CAD build for the part. Positions are in the model's coordinates, mm. A direction names the side the tool comes from. Give positions to 0.01 mm unless a question says otherwise; leave off trailing zeros. Write each loop counter-clockwise with the first axis right and the second up, starting at its lowest first coordinate (ties: lowest second). Pieces come first, ordered by that corner, then holes. Notation, with made-up numbers: (-27.5, 61) - (11.5, 61) arc R22 cw to (11.5, 69) - close; hole circle Ø9 at (16, 21.25). An arc over 180 degrees is marked (long way). Answer as a JSON object with one key per item and string values.
from build123d import *

# Parameters (mm, degrees)
SKETCH1_R           = 1.5
SKETCH1_R_2         = 6.25
SKETCH1_R_3         = 2.55
SKETCH1_R_4         = 4.25
BOSS_EXTRUDE1_DEPTH = 12
SKETCH2_R           = 9
CUT_EXTRUDE1_DEPTH  = 2
SKETCH3_R           = 1.5
CUT_EXTRUDE2_DEPTH  = 210.485083001
SKETCH4_R           = 3.25
CUT_EXTRUDE3_DEPTH  = 25
FILLET1_R           = 2


with BuildPart() as part:
    # Sketch1 → Boss-Extrude1 (new body)
    with BuildSketch(Plane(origin=(0, 0, 0), x_dir=(1, 0, 0), z_dir=(0, 1, 0))):
        with BuildLine():
            Line((55, 122), (55, 117))
            Line((55, 117), (0, 117))
            Line((0, 117), (0, 0))
            Line((0, 0), (30, 0))
            Line((30, 0), (30, 1))
            Line((30, 1), (72.5, 1))
            Line((72.5, 1), (72.5, -39))
            Line((72.5, -39), (82.5, -39))
            Line((82.5, -39), (82.5, 40))
            ThreePointArc((82.5, 40), (85, 89.172897463), (87.5, 40))
            Line((87.5, 40), (87.5, -39))
            Line((87.5, -39), (97.5, -39))
            Line((97.5, -39), (97.5, 1))
            Line((97.5, 1), (140, 1))
            Line((140, 1), (140, 0))
            Line((140, 0), (170, 0))
            Line((170, 0), (170, 117))
            Line((170, 117), (115, 117))
            Line((115, 117), (115, 122))
            Line((115, 122), (55, 122))
        make_face()
        with Locations(Location((65, 116, 0), (0, 0, 270))):
            Circle(SKETCH1_R, mode=Mode.SUBTRACT)
        with Locations(Location((105, 116, 0), (0, 0, 90))):
            Circle(SKETCH1_R, mode=Mode.SUBTRACT)
        with Locations(Location((45, 113.5, 0), (0, 0, 270))):
            Circle(SKETCH1_R, mode=Mode.SUBTRACT)
        with Locations(Location((15, 113.5, 0), (0, 0, 270))):
            Circle(SKETCH1_R, mode=Mode.SUBTRACT)
        with Locations(Location((155, 113.5, 0), (0, 0, 90))):
            Circle(SKETCH1_R, mode=Mode.SUBTRACT)
        with Locations(Location((125, 113.5, 0), (0, 0, 90))):
            Circle(SKETCH1_R, mode=Mode.SUBTRACT)
        with Locations(Location((15, 30, 0), (0, 0, 270))):
            Circle(SKETCH1_R_2, mode=Mode.SUBTRACT)
        with Locations(Location((155, 30, 0), (0, 0, 90))):
            Circle(SKETCH1_R_2, mode=Mode.SUBTRACT)
        with Locations(Location((5, 51, 0), (0, 0, 270))):
            Circle(SKETCH1_R, mode=Mode.SUBTRACT)
        with Locations(Location((25, 51, 0), (0, 0, 90))):
            Circle(SKETCH1_R, mode=Mode.SUBTRACT)
        with Locations(Location((45, 11, 0), (0, 0, 270))):
            Circle(SKETCH1_R_3, mode=Mode.SUBTRACT)
        with Locations(Location((55, 11, 0), (0, 0, 270))):
            Circle(SKETCH1_R_3, mode=Mode.SUBTRACT)
        with Locations(Location((45, 21, 0), (0, 0, 270))):
            Circle(SKETCH1_R_3, mode=Mode.SUBTRACT)
        with Locations(Location((55, 21, 0), (0, 0, 270))):
            Circle(SKETCH1_R_3, mode=Mode.SUBTRACT)
        with Locations(Location((125, 11, 0), (0, 0, 90))):
            Circle(SKETCH1_R_3, mode=Mode.SUBTRACT)
        with Locations(Location((125, 21, 0), (0, 0, 90))):
            Circle(SKETCH1_R_3, mode=Mode.SUBTRACT)
        with Locations(Location((115, 21, 0), (0, 0, 90))):
            Circle(SKETCH1_R_3, mode=Mode.SUBTRACT)
        with Locations(Location((115, 11, 0), (0, 0, 90))):
            Circle(SKETCH1_R_3, mode=Mode.SUBTRACT)
        with Locations(Location((155, 10, 0), (0, 0, 270))):
            Circle(SKETCH1_R_4, mode=Mode.SUBTRACT)
        with Locations(Location((15, 10, 0), (0, 0, 90))):
            Circle(SKETCH1_R_4, mode=Mode.SUBTRACT)
        with Locations(Location((85, 116, 0), (0, 0, 270))):
            Circle(SKETCH1_R, mode=Mode.SUBTRACT)
        with BuildLine():
            ThreePointArc((71.205621302, 99.178418183), (58.624917062, 90.897980402), (50.344479281, 78.317276162))
            ThreePointArc((50.344479281, 78.317276162), (52.301959095, 73.771038951), (56.848196306, 75.728518765))
            ThreePointArc((56.848196306, 75.728518765), (63.57466453, 85.948232933), (73.794378698, 92.674701158))
            ThreePointArc((73.794378698, 92.674701158), (75.751858513, 97.220938368), (71.205621302, 99.178418183))
        make_face(mode=Mode.SUBTRACT)
        with BuildLine():
            ThreePointArc((98.794378698, 99.178418183), (111.375082938, 90.897980402), (119.655520719, 78.317276162))
            ThreePointArc((119.655520719, 78.317276162), (117.698040905, 73.771038951), (113.151803694, 75.728518765))
            ThreePointArc((113.151803694, 75.728518765), (106.42533547, 85.948232933), (96.205621302, 92.674701158))
            ThreePointArc((96.205621302, 92.674701158), (94.248141487, 97.220938368), (98.794378698, 99.178418183))
        make_face(mode=Mode.SUBTRACT)
        with BuildLine():
            ThreePointArc((71.205621302, 29.867376744), (58.624917062, 38.147814525), (50.344479281, 50.728518765))
            ThreePointArc((50.344479281, 50.728518765), (52.301959095, 55.274755976), (56.848196306, 53.317276162))
            ThreePointArc((56.848196306, 53.317276162), (63.57466453, 43.097561993), (73.794378698, 36.371093769))
            ThreePointArc((73.794378698, 36.371093769), (75.751858513, 31.824856558), (71.205621302, 29.867376744))
        make_face(mode=Mode.SUBTRACT)
        with BuildLine():
            ThreePointArc((98.794378698, 29.867376744), (111.375082938, 38.147814525), (119.655520719, 50.728518765))
            ThreePointArc((119.655520719, 50.728518765), (117.698040905, 55.274755976), (113.151803694, 53.317276162))
            ThreePointArc((113.151803694, 53.317276162), (106.42533547, 43.097561993), (96.205621302, 36.371093769))
            ThreePointArc((96.205621302, 36.371093769), (94.248141487, 31.824856558), (98.794378698, 29.867376744))
        make_face(mode=Mode.SUBTRACT)
    extrude(amount=BOSS_EXTRUDE1_DEPTH)

    # Sketch2 → Cut-Extrude1 (cut)
    with BuildSketch(Plane(origin=(0, 12, 0), x_dir=(1, 0, 0), z_dir=(0, 1, 0))):
        with Locations(Location((141.55, 64.522897463, 0), (0, 0, 270))):
            Circle(SKETCH2_R)
    extrude(amount=-CUT_EXTRUDE1_DEPTH, mode=Mode.SUBTRACT)

    # Sketch3 → Cut-Extrude2 (cut, through all)
    with BuildSketch(Plane(origin=(0, 10, 0), x_dir=(1, 0, 0), z_dir=(0, 1, 0))):
        with Locations(Location((141.55, 64.522897463, 0), (0, 0, 270))):
            Circle(SKETCH3_R)
    extrude(amount=-CUT_EXTRUDE2_DEPTH, mode=Mode.SUBTRACT)

    # Sketch4 → Cut-Extrude3 (cut)
    with BuildSketch(Plane.ZY.offset(-72.5)):
        with Locations((29, 6)):
            Circle(SKETCH4_R)
    extrude(amount=-CUT_EXTRUDE3_DEPTH, mode=Mode.SUBTRACT)

    # Fillet1
    # the kernel refuses this fillet: 2 mm, written as the material it adds along each edge
    with BuildSketch(Plane(origin=(72.5, 0, -1), x_dir=(-1, 0, 0), z_dir=(0, 1, 0))) as fillet1_piece_1:
        with BuildLine():
            CenterArc((FILLET1_R, FILLET1_R), FILLET1_R, 180, 90)
            Line((0, FILLET1_R), (0, 0))
            Line((0, 0), (FILLET1_R, 0))
        make_face()
    extrude(amount=12)
    with BuildSketch(Plane(origin=(97.5, 0, -1), x_dir=(1, 0, 0), z_dir=(0, 1, 0))) as fillet1_piece_2:
        with BuildLine():
            CenterArc((FILLET1_R, -FILLET1_R), FILLET1_R, 90, 90)
            Line((0, -FILLET1_R), (0, 0))
            Line((0, 0), (FILLET1_R, 0))
        make_face()
    extrude(amount=12)
    # the kernel refuses this fillet: 2 mm, written as the material it takes off along each edge
    with BuildSketch(Plane(origin=(170, -5, 0), x_dir=(0, 0, -1), z_dir=(0, 1, 0)), Plane(origin=(97.5, -5, 39), x_dir=(0, 0, -1), z_dir=(0, 1, 0))) as fillet1_2_piece_1:
        with BuildLine():
            CenterArc((FILLET1_R, FILLET1_R), FILLET1_R, 180, 90)
            Line((0, FILLET1_R), (0, 0))
            Line((0, 0), (FILLET1_R, 0))
        make_face()
    extrude(amount=22, mode=Mode.SUBTRACT)
    with BuildSketch(Plane(origin=(140, -4.330127019, 0), x_dir=(1, 0, 0), z_dir=(0, 1, 0))) as fillet1_2_piece_2:
        with BuildLine():
            CenterArc((1.732050808, 2), FILLET1_R, 210, 60)
            Line((0, 1), (0, 0))
            Line((0, 0), (1.732050808, 0))
        make_face()
    extrude(amount=20.660254038, mode=Mode.SUBTRACT)
    with BuildSketch(Plane(origin=(72.5, -5, 39), x_dir=(0, 0, -1), z_dir=(0, 1, 0)), Plane(origin=(0, -5, 0), x_dir=(0, 0, -1), z_dir=(0, 1, 0))) as fillet1_2_piece_3:
        with BuildLine():
            CenterArc((FILLET1_R, -FILLET1_R), FILLET1_R, 90, 90)
            Line((0, -FILLET1_R), (0, 0))
            Line((0, 0), (FILLET1_R, 0))
        make_face()
    extrude(amount=22, mode=Mode.SUBTRACT)
    with BuildSketch(Plane(origin=(30, -4.330127019, 0), x_dir=(-1, 0, 0), z_dir=(0, 1, 0))) as fillet1_2_piece_4:
        with BuildLine():
            CenterArc((1.732050808, -2), FILLET1_R, 90, 60)
            Line((0, -1), (0, 0))
            Line((0, 0), (1.732050808, 0))
        make_face()
    extrude(amount=20.660254038, mode=Mode.SUBTRACT)


solid = part.part
(1) Flat gauge pins, fed straight in: P1, Ø1, axis at x = 147, y = 4, coming from the +Z side; P2, Ø9, axis at x = 142, z = -64.5, coming from the +Y side; P3, Ø3.5, axis at x = 119.5, y = 6.5, coming from the +Z side. Where does each tip first touch, or does it go through?
Answer key:
{"P1": "stops at z = 0", "P2": "stops at y = 10", "P3": "stops at z = -1"}
(2) Saw through at D-D, the plane z = -26.5. Give the cut face in (x, y), and give its area (3 significant figures).
Answer key:
{"outline": "(0, 0) - (9.82, 0) - (9.82, 12) - (0, 12) - close; (20.18, 0) - (82.5, 0) - (82.5, 12) - (20.18, 12) - close; (87.5, 0) - (149.82, 0) - (149.82, 12) - (87.5, 12) - close; (160.18, 0) - (170, 0) - (170, 12) - (160.18, 12) - close", "area": "1,730 mm²"}
(3) Saw through at C-C, the plane x = 130.5. Give the cut face in (y, z).
Answer key:
{"outline": "(0, -117) - (12, -117) - (12, -1) - (0, -1) - close"}
(4) Saw through at A-A, the plane z = 22. Give the cut face in (x, y).
Answer key:
{"outline": "(72.5, 0) - (82.5, 0) - (82.5, 12) - (72.5, 12) - close; (87.5, 0) - (97.5, 0) - (97.5, 12) - (87.5, 12) - close"}
(5) Pull direction Z, two halves, no side cores. Call faces 1 (the face through (55, 6, -120)), 2 (the face through (85, 6, -122)), 3 (the face through (15, 6, 0)), 4 (the face through (106.547, 5.916, -85.826)): pulls with the +Z half, pulls with the -Z half, needs draft (parallel to the pull), parting line crosses it, or undercut.
Answer key:
{"face 1": "needs draft", "face 2": "pulls with the -Z half", "face 3": "pulls with the +Z half", "face 4": "undercut"}
(6) Saw through at B-B, the plane z = -47. Give the cut face in (x, y), and give its area (3 significant figures).
Answer key:
{"outline": "(0, 0) - (52.07, 0) - (52.07, 12) - (0, 12) - close; (60.28, 0) - (67.66, 0) - (67.66, 12) - (60.28, 12) - close; (102.34, 0) - (109.72, 0) - (109.72, 12) - (102.34, 12) - close; (117.93, 0) - (170, 0) - (170, 12) - (117.93, 12) - close", "area": "1,430 mm²"}
(7) Probe L1, parallel to X at y = 9.25, z = -113.5; L2, parallel to X at y = 3.5, z = -116; L3, parallel to X at y = 6.25, z = -21. List the from-to ranges inside material, lowest first. Write a range as [from, to].
Answer key:
{"L1": "x = [0, 13.5], [16.5, 43.5], [46.5, 123.5], [126.5, 153.5], [156.5, 170]", "L2": "x = [0, 63.5], [66.5, 83.5], [86.5, 103.5], [106.5, 170]", "L3": "x = [0, 42.45], [47.55, 52.45], [57.55, 82.5], [87.5, 112.45], [117.55, 122.45], [127.55, 170]"}
(8) 3-axis set-ups, long thin cutter, end or side, ignore diameter. For faces 5 (the face through (58.775, 5.916, -37.998)), 6 (the face through (50, 6, -1)), 7 (the face through (28, 6, -117)): which of +Z, -Z, +X, -X, +Y, -Y reach the whole face in a straight line?
Answer key:
{"face 5": "+Y, -Y", "face 6": "+Z, +Y, -Y", "face 7": "-Z, -X, +Y, -Y"}
